The model under review builds one solid part; all positions refer to its coordinate system, in mm. A direction names the side the tool comes from. Give positions to 0.01 mm unless a question says otherwise; leave off trailing zeros. Loops run counter-clockwise (first coordinate to the right, second up) from the corner with the lowest first, then second, coordinate; pieces in that order, holes last. Notation, with made-up numbers: (74, 63.5) -> (114, 63.5) arc R20 ccw to (114, 74.5) -> close; hole circle Ø11 at (28, 35). An arc over 180 degrees is marked (long way). Write each question's results on one line, items separated by ' | '. Start each with the question number.
Q1. We need section D-D (x = -43). Write out the cut boundary in (y, z), plus the area to 3 significant figures.
Q2. Insertion check: pin 1 Ø1.5 at (y, z) = (33.5, 2.5) entering from -X; pin 2 Ø0.8 at (x, z) = (-39.5, 1.5) entering from -Y; pin 3 Ø1 at (x, z) = (-38.5, 0.5) entering from +Y. Each pin has a flat end and moves straight along its axis. Give the tip position at first contact, or say it passes through.
Q3. We need section A-A (x = -23.5). Write out the cut boundary in (y, z), plus the area to 3 significant figures.
Q4. Mouldability with a two-part tool opening along Y and no side actions: class faces 5 (the face through (-43.63, 13.8, 2.46)), 6 (the face through (-26.705, 13, 2)), 7 (the face through (-33.788, 9, 2)) as released by +Y, released by -Y, zero draft, split by the parting line, or undercut.
Q5. Machinability: for faces 1 (the face through (-24.165, 35, 2)), 2 (the face through (-28.963, 18, 2)), 3 (the face through (-21.625, 26, 2)), 4 (the face through (-38.585, 35, 2)), which of the approach directions +Z, -Z, +X, -X, +Y, -Y give a long, thin tool a straight path to every point of the face, cutting with its end or side? Answer none if there is none.
Q6. We need section C-C (y = 32). Write out the cut boundary in (x, z).
Q7. Wall thickness on L1, parallel to X at y = 5, z = 1.05; L2, parallel to Y at x = -29.75, z = 3.75; L3, parallel to X at y = 17.5, z = 2.75: over which ranges is each line inside the solid? List them lowest first. Write a range as [from, to].
from build123d import *

# Parameters (mm, degrees)
SKETCH1_R           = 1.955
BOSS_EXTRUDE1_DEPTH = 5


with BuildPart() as part:
    # Sketch1 → Boss-Extrude1 (new body)
    with BuildSketch(Plane.XY):
        with BuildLine():
            Line((-46.205346306, 6.069), (-46.205346306, 0))
            Line((-46.205346306, 0), (-40.278346306, 0))
            Line((-40.278346306, 0), (-40.278346306, 6.209))
            Line((-40.278346306, 6.209), (-33.788346306, 6.209))
            Line((-33.788346306, 6.209), (-33.788346306, 11.008))
            Line((-33.788346306, 11.008), (-36.045346306, 11.008))
            Line((-36.045346306, 11.008), (-36.045346306, 15.241))
            Line((-36.045346306, 15.241), (-33.787346306, 15.241))
            Line((-33.787346306, 15.241), (-33.787346306, 20.018965401))
            Line((-33.787346306, 20.018965401), (-31.375346306, 20.018965401))
            Line((-31.375346306, 20.018965401), (-28.963346306, 20.018965401))
            Line((-28.963346306, 20.018965401), (-28.963346306, 15.241))
            Line((-28.963346306, 15.241), (-26.705346306, 15.241))
            Line((-26.705346306, 15.241), (-26.705346306, 11.008))
            Line((-26.705346306, 11.008), (-28.962346306, 11.008))
            Line((-28.962346306, 11.008), (-28.962346306, 6.209))
            Line((-28.962346306, 6.209), (-22.472346306, 6.209))
            Line((-22.472346306, 6.209), (-22.472346306, 0))
            Line((-22.472346306, 0), (-16.545346306, 0))
            Line((-16.545346306, 0), (-16.545346306, 6.069))
            Line((-16.545346306, 6.069), (-21.625346306, 21.309))
            Line((-21.625346306, 21.309), (-21.625346306, 31.309))
            Line((-21.625346306, 31.309), (-24.165346306, 31.309))
            Line((-24.165346306, 31.309), (-24.165346306, 38.082))
            Line((-24.165346306, 38.082), (-21.625346306, 38.082))
            ThreePointArc((-21.625346306, 38.082), (-23.900792185, 42.177151256), (-27.90009545, 44.61712895))
            Line((-27.90009545, 44.61712895), (-31.366233796, 44.61712895))
            Line((-31.366233796, 44.61712895), (-31.384458817, 44.61712895))
            Line((-31.384458817, 44.61712895), (-34.850597163, 44.61712895))
            ThreePointArc((-34.850597163, 44.61712895), (-38.849900428, 42.177151256), (-41.125346306, 38.082))
            Line((-41.125346306, 38.082), (-38.585346306, 38.082))
            Line((-38.585346306, 38.082), (-38.585346306, 31.309))
            Line((-38.585346306, 31.309), (-41.125346306, 31.309))
            Line((-41.125346306, 31.309), (-41.125346306, 21.309))
            Line((-41.125346306, 21.309), (-46.205346306, 6.069))
        make_face()
        with Locations((-31.375346306, 34.658965401)):
            Circle(SKETCH1_R, mode=Mode.SUBTRACT)
    extrude(amount=BOSS_EXTRUDE1_DEPTH)


solid = part.part
Output:
1) outline: (0, 0) -> (15.69, 0) -> (15.69, 5) -> (0, 5) -> close | area: 78.4 mm2
2) pin 1: x = -38.59 | pin 2: y = 6.21 | pin 3: y = 42.96
3) outline: (6.21, 0) -> (31.31, 0) -> (31.31, 5) -> (6.21, 5) -> close; (38.08, 0) -> (41.73, 0) -> (41.73, 5) -> (38.08, 5) -> close | area: 144 mm2
4) face 5: released by +Y | face 6: undercut | face 7: zero draft
5) face 1: +Z, -Z, +X | face 2: +Z, -Z, -Y | face 3: +Z, -Z, +X, +Y | face 4: +Z, -Z, -X
6) outline: (-38.59, 0) -> (-24.17, 0) -> (-24.17, 5) -> (-38.59, 5) -> close
7) L1: [-46.21, -40.28], [-22.47, -16.55] | L2: [20.02, 33.57], [35.75, 44.62] | L3: [-42.4, -33.79], [-28.96, -20.36]
